Geometry: final body of the model. Coordinates: model frame, mm. A direction names the side the tool comes from. Round coordinates to 2 decimals unless told otherwise and drop trailing zeros. Loops run counter-clockwise (first coordinate to the right, second up) from the corner with the lowest first, then second, coordinate; pieces in that order, holes last. Notation, with made-up numbers: (5, 83) - (51, 83) arc R12 cw to (51, 92) - close; hole circle Ø8 at (70.25, 44.25). An arc over 180 degrees is marked (long way). Answer as a JSON object with one key per item and string values. Group by question number.
Item 1: Section B-B (z = 2.5). Return the cut outline in (x, y).
Item 2: Section C-C (y = -1.75). Return the cut outline in (x, z).
Item 3: Section A-A (x = -6). Return the cut outline in (y, z), plus the area to 3 significant figures.
Item 4: First-contact query: pin 1 (5 mm diameter, centred on x = -2.5, z = 4.5, fed in from +Y); pin 2 (1 mm diameter, centred on y = -2.5, z = -3, fed in from -X); pin 3 (2.5 mm diameter, centred on x = -16.5, z = 0, fed in from -Y); pin 4 (0.7 mm diameter, centred on x = 13.5, y = -1.5, fed in from +Z). Flat tips, straight axial feed; report the tip coordinate or a pass-through.
Item 5: Section D-D (x = 16.5). Return the cut outline in (y, z), plus the area to 3 significant figures.
Item 6: Line query: line 1 (Z direction, x = -6, y = -2.1); line 2 (X direction, y = -2.55, z = -0.25); line 3 (X direction, y = -4, z = 0.75). Output: solid intervals per line, ascending.
Item 7: Draft query along Z for faces 1 (the face through (-19.75, -2.46, 0.11)), 2 (the face through (-3.14, -2.71, 0.9)), 3 (the face through (11.9, -2.46, -6.93)), 4 (the face through (13, -2, 2)). Return one class per face: released by +Z, released by -Z, zero draft, split by the parting line, or undercut.
Item 8: Reachability of faces 5 (the face through (-12.5, -2, -4)), 6 (the face through (-13, -2, 2)), 7 (the face through (14.9, -2.5, -1.2)) from +Z, -Z, +X, -X, +Y, -Y: full face, straight path, thin tool, end or side. Return the list, or none.
```python
from build123d import *

# Parameters (mm, degrees)
F0_R     = 2
F0_R_2   = 4
F1_DEPTH = 5
F0_R_3   = 3
F2_DEPTH = 5.5


with BuildPart() as f1:
    # F0 (on Front) → F1 (new body)
    with BuildSketch(Plane.XZ):
        with BuildLine():
            Line((14.2, -2), (13.938262, -2))
            ThreePointArc((13.938262, -2), (17.557557, -3.073121), (19.75, 0))
            ThreePointArc((19.75, 0), (17.557557, 3.073121), (13.938262, 2))
            Line((13.938262, 2), (14.2, 2))
            Line((14.2, 2), (14.2, -2))
        make_face()
        with Locations((16.5, 0)):
            Circle(F0_R, mode=Mode.SUBTRACT)
        with BuildLine():
            ThreePointArc((13.938262, 2), (13.25, 0), (13.938262, -2))
            Line((13.938262, -2), (14.2, -2))
            Line((14.2, -2), (14.2, 2))
            Line((14.2, 2), (13.938262, 2))
        make_face()
        with BuildLine():
            Line((12.5, 2), (12.5, -2))
            Line((12.5, -2), (13.938262, -2))
            ThreePointArc((13.938262, -2), (13.25, 0), (13.938262, 2))
            Line((13.938262, 2), (12.5, 2))
        make_face()
        with BuildLine():
            ThreePointArc((-13.938262, 2), (-19.75, 0), (-13.938262, -2))
            Line((-13.938262, -2), (-14.2, -2))
            Line((-14.2, -2), (-14.2, 2))
            Line((-14.2, 2), (-13.938262, 2))
        make_face()
        with Locations((-16.5, 0)):
            Circle(F0_R, mode=Mode.SUBTRACT)
        with BuildLine():
            Line((-14.2, -2), (-13.938262, -2))
            ThreePointArc((-13.938262, -2), (-13.426879, -1.057557), (-13.25, 0))
            ThreePointArc((-13.25, 0), (-13.426879, 1.057557), (-13.938262, 2))
            Line((-13.938262, 2), (-14.2, 2))
            Line((-14.2, 2), (-14.2, -2))
        make_face()
        with BuildLine():
            Line((-13.938262, -2), (-12.5, -2))
            Line((-12.5, -2), (-12.5, 2))
            Line((-12.5, 2), (-13.938262, 2))
            ThreePointArc((-13.938262, 2), (-13.426879, 1.057557), (-13.25, 0))
            ThreePointArc((-13.25, 0), (-13.426879, -1.057557), (-13.938262, -2))
        make_face()
        with BuildLine():
            Line((-10.5, -7.5), (10.5, -7.5))
            ThreePointArc((10.5, -7.5), (11.914214, -6.914214), (12.5, -5.5))
            Line((12.5, -5.5), (12.5, -2))
            Line((12.5, -2), (12.5, 2))
            Line((12.5, 2), (12.5, 5.5))
            ThreePointArc((12.5, 5.5), (11.914214, 6.914214), (10.5, 7.5))
            Line((10.5, 7.5), (-10.5, 7.5))
            ThreePointArc((-10.5, 7.5), (-11.914214, 6.914214), (-12.5, 5.5))
            Line((-12.5, 5.5), (-12.5, 2))
            Line((-12.5, 2), (-12.5, -2))
            Line((-12.5, -2), (-12.5, -5.5))
            ThreePointArc((-12.5, -5.5), (-11.914214, -6.914214), (-10.5, -7.5))
        make_face()
        with Locations((-6, 0)):
            Circle(F0_R_2, mode=Mode.SUBTRACT)
        with Locations((6, 0)):
            Circle(F0_R_2, mode=Mode.SUBTRACT)
    extrude(amount=F1_DEPTH)

    # F0 (on Front) → F2 (join)
    with BuildSketch(Plane.XZ):
        with Locations((-6, 0)):
            Circle(F0_R_2)
        with Locations((-6, 0)):
            Circle(F0_R_3, mode=Mode.SUBTRACT)
        with Locations((6, 0)):
            Circle(F0_R_2)
        with Locations((6, 0)):
            Circle(F0_R_3, mode=Mode.SUBTRACT)
    extrude(amount=F2_DEPTH)


solid = f1.part
```
Values:
{
 "1": {"outline": "(-18.58, -5) - (-14.42, -5) - (-14.42, 0) - (-18.58, 0) - close; (-12.5, -5) - (-9.12, -5) - (-9.12, -5.5) - (-7.66, -5.5) - (-7.66, 0) - (-12.5, 0) - close; (-4.34, -5.5) - (-2.88, -5.5) - (-2.88, -5) - (2.88, -5) - (2.88, -5.5) - (4.34, -5.5) - (4.34, 0) - (-4.34, 0) - close; (7.66, -5.5) - (9.12, -5.5) - (9.12, -5) - (12.5, -5) - (12.5, 0) - (7.66, 0) - close; (14.42, -5) - (18.58, -5) - (18.58, 0) - (14.42, 0) - close"},
 "2": {"outline": "(-13.94, -2) - (-12.5, -2) - (-12.5, -5.5) arc R2 ccw to (-10.5, -7.5) - (10.5, -7.5) arc R2 ccw to (12.5, -5.5) - (12.5, -2) - (13.94, -2) arc R3.25 ccw (long way) to (13.94, 2) - (12.5, 2) - (12.5, 5.5) arc R2 ccw to (10.5, 7.5) - (-10.5, 7.5) arc R2 ccw to (-12.5, 5.5) - (-12.5, 2) - (-13.94, 2) arc R3.25 ccw (long way) to start; hole circle Ø4 at (-16.5, 0); hole circle Ø6 at (-6, 0); hole circle Ø6 at (6, 0); hole circle Ø4 at (16.5, 0)"},
 "3": {"outline": "(-5.5, -4) - (-5, -4) - (-5, -7.5) - (0, -7.5) - (0, -3) - (-5.5, -3) - close; (-5.5, 3) - (0, 3) - (0, 7.5) - (-5, 7.5) - (-5, 4) - (-5.5, 4) - close", "area": "46.0 mm^2"},
 "4": {"pin 1": "stops at y = 0", "pin 2": "stops at x = -18.58", "pin 3": "passes through", "pin 4": "stops at z = 2"},
 "5": {"outline": "(-5, -3.25) - (0, -3.25) - (0, -2) - (-5, -2) - close; (-5, 2) - (0, 2) - (0, 3.25) - (-5, 3.25) - close", "area": "12.5 mm^2"},
 "6": {"line 1": "z = -7.5 to -3, 3 to 7.5", "line 2": "x = -19.74 to -18.48, -14.52 to -8.99, -3.01 to 3.01, 8.99 to 14.52, 18.48 to 19.74", "line 3": "x = -19.66 to -18.35, -14.65 to -8.9, -3.1 to 3.1, 8.9 to 14.65, 18.35 to 19.66"},
 "7": {"face 1": "split by the parting line", "face 2": "undercut", "face 3": "released by -Z", "face 4": "released by +Z"},
 "8": {"face 5": "-Z, +Y, -Y", "face 6": "+Z, +Y, -Y", "face 7": "+Y, -Y"}
}
